Here's the drawing with two shaded views (mm, measured from the low corner). I have some questions. Coordinates: 2 decimals unless noted, no trailing zeros. Order: outer loops, then holes, each group sorted by start corner. A loop starts at its lowest first (then second) coordinate and runs counter-clockwise, first axis right, second up. Notation, with made-up numbers: (88.25, 21.5) - (125.25, 21.5) arc R33 cw to (125.25, 56.5) - close; hole circle Ø6 at (68.5, -3). An arc over 180 degrees is marked (long way). Answer as CSV lines item,"result". Start each with the question number.
1. I want a section at C-C, the plane x = 70.2. List the corners of the cut face in (y, z) for me.
2. I want a section at D-D, the plane y = 1.5. List the corners of the cut face in (x, z) for me.
3. I need wall thicknesses on probe 1 along X at (y, z) = (1.7, 5); probe 2 along Z at (x, y) = (91, 0.4); probe 3 along X at (y, z) = (1.35, 24.2). Which ranges of each line are inside material? Lowest first, please.
4. For pin 1 (3 mm diameter, centred on x = 91, z = 47, fed in from +Y), with a flat end and sliding along its axis, tell me the tip position at first contact or that it passes through.
5. I want a section at A-A, the plane x = 5. List the corners of the cut face in (y, z) for me, and give its area (3 significant figures).
6. I want a section at B-B, the plane z = 47. List the corners of the cut face in (x, y) for me.
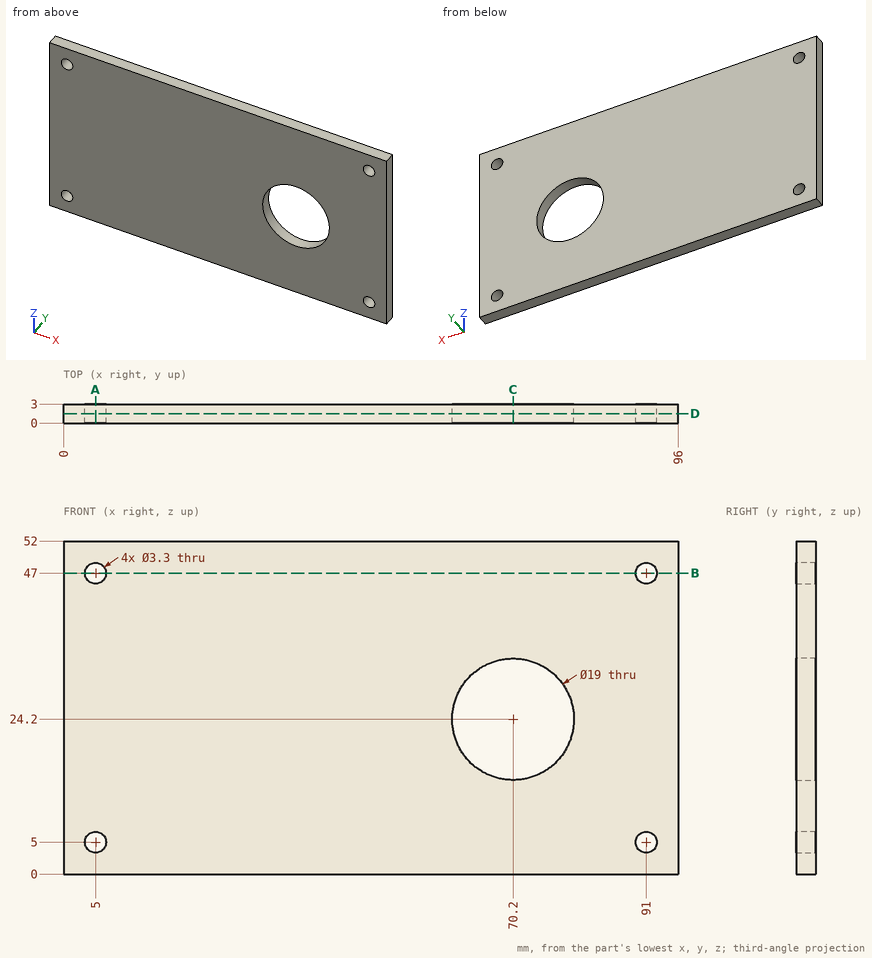
Solved:
1,outline,"(0, 0) - (3, 0) - (3, 14.7) - (0, 14.7) - close; (0, 33.7) - (3, 33.7) - (3, 52) - (0, 52) - close"
2,outline,"(0, 0) - (96, 0) - (96, 52) - (0, 52) - close; hole circle Ø3.3 at (5, 5); hole circle Ø3.3 at (5, 47); hole circle Ø19 at (70.2, 24.2); hole circle Ø3.3 at (91, 5); hole circle Ø3.3 at (91, 47)"
3,probe 1,"x = 0 to 3.35, 6.65 to 89.35, 92.65 to 96"
3,probe 2,"z = 0 to 3.35, 6.65 to 45.35, 48.65 to 52"
3,probe 3,"x = 0 to 60.7, 79.7 to 96"
4,pin 1,"passes through"
5,outline,"(0, 0) - (3, 0) - (3, 3.35) - (0, 3.35) - close; (0, 6.65) - (3, 6.65) - (3, 45.35) - (0, 45.35) - close; (0, 48.65) - (3, 48.65) - (3, 52) - (0, 52) - close"
5,area,"136 mm2"
6,outline,"(0, 0) - (3.35, 0) - (3.35, 3) - (0, 3) - close; (6.65, 0) - (89.35, 0) - (89.35, 3) - (6.65, 3) - close; (92.65, 0) - (96, 0) - (96, 3) - (92.65, 3) - close"
